Check sheet for the modelled part. Datum: model origin and axes. Units: mm. Give positions to 0.01 mm unless a question says otherwise; leave off trailing zeros. Loops run counter-clockwise (first coordinate to the right, second up) from the corner with the lowest first, then second, coordinate; pieces in that order, holes last. Notation, with made-up numbers: (36, 41.5) -> (72, 41.5) arc R34 ccw to (72, 79.5) -> close; hole circle Ø6 at (66, -2.5). An arc over 180 degrees is marked (long way). Answer as CSV lines item,"result". Start each with the question number.
(1) Section check C-C on z = -0.2. Enter the section's corners in (x, y).
(2) Release check for a two-part mould opening along Y. For faces 1 (the face through (3.434, 1.081, -0.592)), 2 (the face through (-0.867, -3.905, -0.186)), 3 (the face through (2, 2, 0)), 4 (the face through (3, 0, 0.8)) record: pulls with the +Y half, pulls with the -Y half, needs draft (parallel to the pull), parting line crosses it, or undercut.
(3) Material ranges on line 1 (Y direction, x = 0, z = 0.25); line 2 (Y direction, x = 0, z = -0.6); line 3 (Z direction, x = 2.5, y = -1.5), recorded low to high. Write a range as from..to.
(4) Section check A-A on x = 0. Enter the section's corners in (y, z), plus the area to 3 significant figures.
(5) Section check D-D on y = 3.5. Enter the section's corners in (x, z), plus the area to 3 significant figures.
(6) Gauge pin test, flat ends, axial feed: pin 1 Ø4 at (x, y) = (-2.5, 1) entering from -Z; pin 2 Ø2 at (x, y) = (-1, 1.5) entering from -Z; pin 3 Ø4.5 at (x, y) = (0, 0) entering from +Z. Record the tip position at first contact, or that the pin passes through.
Autodesk Inventor part; units mm, degrees
ref_plane "YZ Plane" through (0, 0, 0) normal (1, 0, 0) x (0, 1, 0)
ref_plane "XZ Plane" through (0, 0, 0) normal (0, 1, 0) x (-1, 0, 0)
ref_plane "XY Plane" through (0, 0, 0) normal (0, 0, 1) x (1, 0, 0)
sketch "Sketch1" plane through (0, 0, 0) normal (0, 0, 1) x (1, 0, 0)
  circle A0 centre (0, 0) radius 4
  dimension "d0" = 8
extrude "Extrusion1" add sketch "Sketch1" along normal blind 0.8
sketch "Sketch2" plane through (0, 0, 0) normal (0, 0, 1) x (1, 0, 0)
  circle A0 centre (0, 0) radius 3.6
  circle A1 centre (0, 0) radius 4
  dimension "d3" = 7.2
extrude "Extrusion2" add sketch "Sketch2" against normal blind 1.2
sketch "Sketch3" plane through (0, 0, 0.8) normal (0, 0, 1) x (1, 0, 0)
  point P0 (0, 0)
hole "Hole1" at (0, 0, 0.8) direction (0, 0, -1) diameter 5.2 end through all
properties part number "LabyrinthSealOuter"
Working result:
1,outline,"circle Ø8 at (0, 0); hole circle Ø7.2 at (0, 0)"
2,face 1,"undercut"
2,face 2,"parting line crosses it"
2,face 3,"undercut"
2,face 4,"needs draft"
3,line 1,"y = -4..-2.6, 2.6..4"
3,line 2,"y = -4..-3.6, 3.6..4"
3,line 3,"z = 0..0.8"
4,outline,"(-4, -1.2) -> (-3.6, -1.2) -> (-3.6, 0) -> (-2.6, 0) -> (-2.6, 0.8) -> (-4, 0.8) -> close; (2.6, 0) -> (3.6, 0) -> (3.6, -1.2) -> (4, -1.2) -> (4, 0.8) -> (2.6, 0.8) -> close"
4,area,"3.20 mm^2"
5,outline,"(-1.94, -1.2) -> (-0.84, -1.2) -> (-0.84, 0) -> (0.84, 0) -> (0.84, -1.2) -> (1.94, -1.2) -> (1.94, 0.8) -> (-1.94, 0.8) -> close"
5,area,"5.72 mm^2"
6,pin 1,"stops at z = -1.2"
6,pin 2,"stops at z = 0"
6,pin 3,"passes through"
